CAD build for the part. Positions are in the model's coordinates, mm. A direction names the side the tool comes from. Round coordinates to 2 decimals unless told otherwise and drop trailing zeros. Order: outer loops, then holes, each group sorted by start corner. A loop starts at its lowest first (then second) coordinate and runs counter-clockwise, first axis right, second up. Notation, with made-up numbers: (37.25, -25.5) - (75.25, -25.5) arc R17 ccw to (75.25, -0.5) - close; hole circle Ø1 at (30, -33.75). An arc over 180 degrees is marked (long way). Write item = value, one per line.
from build123d import *

# Parameters (mm, degrees)
F0_W     = 177.8
F0_H     = 6.35
F0_W_2   = 165.1
F1_DEPTH = 76.2


with BuildPart() as f1:
    # F0 (on Top) → F1 (new body)
    with BuildSketch(Plane.XY):
        Polygon((508, 0), (-508, 0), (-508, -63.5), (0, -63.5), (405.8161629425, -63.5), (508, -63.5), align=None)
        with Locations((-317.5, -41.275)):
            Rectangle(F0_W, F0_H, mode=Mode.SUBTRACT)
        with Locations((-120.65, -41.275)):
            Rectangle(F0_W_2, F0_H, mode=Mode.SUBTRACT)
        Polygon((-508, -63.5), (-508, 0), (-571.5, -63.5), align=None)
        Polygon((571.5, -63.5), (508, 0), (508, -63.5), align=None)
        Polygon((-508, -69.85), (-508, -63.5), (-571.5, -63.5), (-508, -127), align=None)
        Polygon((571.5, -63.5), (508, -63.5), (508, -88.9), (508.2334558824, -95.2457070805), (508, -95.2542958237), (508, -127), align=None)
        Polygon((508, -88.9), (508, -63.5), (405.8161629425, -63.5), (0, -63.5), (0, -69.85), (-508, -69.85), (-508, -127), (508, -127), (508, -95.2542958237), (-151.7200804854, -119.5251188452), (-151.9535363678, -113.1794117647), align=None)
        Polygon((-457.2, -95.25), (405.8161629425, -63.5), (406.0496188249, -69.8457070805), (-456.9665441176, -101.5957070805), align=None, mode=Mode.SUBTRACT)
        Polygon((456.7191930115, -82.5447314139), (-254, -108.6917902374), (-254.3446927927, -102.351152503), (456.4857730235, -76.2), align=None, mode=Mode.SUBTRACT)
    extrude(amount=F1_DEPTH)


solid = f1.part
(1) Probe line 1 along Y through (x, z) = (-107.5, 35); line 2 along Y through (x, z) = (-37, 44.5); line 3 along Y through (x, z) = (103, 65). List the from-to ranges inside material, lowest first.
Solved:
line_1 = -127 to -117.9, -111.54 to -103.3, -96.95 to -88.74, -82.38 to -69.85, -63.5 to -44.45, -38.1 to 0
line_2 = -127 to -115.3, -108.95 to -100.71, -94.36 to -86.15, -79.79 to -69.85, -63.5 to 0
line_3 = -127 to -110.15, -103.8 to -95.56, -89.2 to -80.99, -74.64 to 0
(2) Band-saw the part on A-A on z = 32.5. Count the separate pieces of the cut face and the enclosed holes in it, plus the area to 4 significant figures.
Solved:
separate_pieces = 1
enclosed_holes = 6
area = 117,500 mm²
(3) Pull direction X, two halves, no side cores. Call faces 3 (the flat face through (96.09, -89.46, 37.57)), 4 (the flat face through (-122, -44.45, 38)), 5 (the flat face through (-540, -95, 38)), 6 (the flat face through (540, -32, 38)): released by +X, released by -X, zero draft, split by the parting line, or undercut.
Solved:
face_3 = undercut
face_4 = undercut
face_5 = released by -X
face_6 = released by +X
(4) Drop flat-ended pins along their axis: pin 1 (1.9 mm diameter, centred on y = -42.5, z = 42, fed in from +X); pin 2 (1.5 mm diameter, centred on y = -100, z = 60, fed in from -X); pin 3 (3 mm diameter, centred on y = -66, z = 46, fed in from -X). Give the stop position or say it passes through.
Solved:
pin_1 = 551.45
pin_2 = -535.75
pin_3 = -570.5
(5) Band-saw the part on B-B on x = 262. List the corners of the cut face in (y, z), plus the area to 3 significant figures.
Solved:
outline = (-127, 0) - (-104.3, 0) - (-104.3, 76.2) - (-127, 76.2) - close; (-97.95, 0) - (-89.71, 0) - (-89.71, 76.2) - (-97.95, 76.2) - close; (-83.36, 0) - (-75.15, 0) - (-75.15, 76.2) - (-83.36, 76.2) - close; (-68.79, 0) - (0, 0) - (0, 76.2) - (-68.79, 76.2) - close
area = 8,220 mm²
(6) Tool access for faces 1 (the flat face through (-258, -63.5, 38)), 2 (the flat face through (-539, -31, 38)): list every direction of +Z, -Z, +X, -X, +Y, -Y with a clear straight run to the whole face (end or side of a thin tool).
Solved:
face_1 = +Z, -Z
face_2 = +Z, -Z, -X, +Y
(7) Band-saw the part on C-C on x = -122. List the corners of the cut face in (y, z), plus the area to 3 significant figures.
Solved:
outline = (-127, 0) - (-118.43, 0) - (-118.43, 76.2) - (-127, 76.2) - close; (-112.08, 0) - (-103.84, 0) - (-103.84, 76.2) - (-112.08, 76.2) - close; (-97.48, 0) - (-89.27, 0) - (-89.27, 76.2) - (-97.48, 76.2) - close; (-82.92, 0) - (-69.85, 0) - (-69.85, 76.2) - (-82.92, 76.2) - close; (-63.5, 0) - (-44.45, 0) - (-44.45, 76.2) - (-63.5, 76.2) - close; (-38.1, 0) - (0, 0) - (0, 76.2) - (-38.1, 76.2) - close
area = 7,260 mm²
(8) Band-saw the part on D-D on y = -17.5. List the corners of the cut face in (x, z).
Solved:
outline = (-525.5, 0) - (525.5, 0) - (525.5, 76.2) - (-525.5, 76.2) - close
